```python
from build123d import *

# Parameters (mm, degrees)
F0_W     = 40
F0_H     = 20
F1_DEPTH = 20
F3_DEPTH = 4
F4_DEPTH = 2
F5_DEPTH = 2
F6_W     = 40
F6_H     = 2
F7_DEPTH = 3


with BuildPart() as f1:
    # F0 (on Top) → F1 (new body)
    with BuildSketch(Plane.XY):
        Rectangle(F0_W, F0_H)
    extrude(amount=F1_DEPTH)

    # F2 (on face) → F3 (join)
    with BuildSketch(Plane.XY.offset(20)):
        with BuildLine():
            Line((-10, -1.5), (-10, 1.5))
            ThreePointArc((-10, 1.5), (-11.5, 0), (-10, -1.5))
        make_face()
        with BuildLine():
            ThreePointArc((-8.5, 0), (-8.9393398282, 1.0606601718), (-10, 1.5))
            Line((-10, 1.5), (-10, -1.5))
            ThreePointArc((-10, -1.5), (-8.9393398282, -1.0606601718), (-8.5, 0))
        make_face()
        with BuildLine():
            Line((10, -1.5), (10, 1.5))
            ThreePointArc((10, 1.5), (8.5, 0), (10, -1.5))
        make_face()
        with BuildLine():
            ThreePointArc((11.5, 0), (11.0606601718, 1.0606601718), (10, 1.5))
            Line((10, 1.5), (10, -1.5))
            ThreePointArc((10, -1.5), (11.0606601718, -1.0606601718), (11.5, 0))
        make_face()
    extrude(amount=F3_DEPTH)

    # F4 (add): a face of the model
    f4_faces = [f1.faces().sort_by_distance(p)[0] for p in [
        (0, -10, 10),
    ]]
    extrude(f4_faces, amount=F4_DEPTH)

    # F5 (add): a face of the model
    f5_faces = [f1.faces().sort_by_distance(p)[0] for p in [
        (0, 10, 10),
    ]]
    extrude(f5_faces, amount=F5_DEPTH)

    # F6 (on face) → F7 (join)
    with BuildSketch(Plane(origin=(0, 0, 0), x_dir=(1, 0, 0), z_dir=(0, 0, -1))):
        with Locations((0, 11)):
            Rectangle(F6_W, F6_H)
        with Locations((0, -11)):
            Rectangle(F6_W, F6_H)
    extrude(amount=F7_DEPTH)


solid = f1.part
```
The model under review builds one solid part; all positions refer to its coordinate system, in mm. A direction names the side the tool comes from. Round coordinates to 2 decimals unless told otherwise and drop trailing zeros. Write each loop counter-clockwise with the first axis right and the second up, starting at its lowest first coordinate (ties: lowest second). Pieces come first, ordered by that corner, then holes. Notation, with made-up numbers: M -35.5,22 L -1.5,22 A16 ccw -1.5,43 Z; hole C 67.25,65 d10. An arc over 180 degrees is marked long. Use CSV: the item, a comma, the result in double quotes. Start each with the question number.
(1) For line 1 along Z through (x, y) = (0.5, 6.75); line 2 along Y through (x, z) = (-11, 20.5), list the stretches that pass through material, from the lowest coordinate up.
(2) We need section A-A, the plane x = 0. State the section outline as (y, z) points, then the cut area to 3 significant figures.
(3) Clearance check with flat-ended pins moving along their axes: P1, Ø3, axis at x = -5, y = 6, coming from the -Z side; P2, Ø8, axis at x = 15, y = 7.5, coming from the +Z side. State where each tip first meets the part, or that it passes through.
(4) Tool access review of faces 4 (the face through (0, -12, 9)), 5 (the face through (0, -10, -1)): name each direction out of +Z, -Z, +X, -X, +Y, -Y from which nothing blocks a thin tool from reaching the whole face with its end or side.
(5) We need section B-B, the plane y = 3. State the section outline as (x, z) points, then the cut area to 3 significant figures.
(6) We need section C-C, the plane x = 11. State the section outline as (y, z) points.
(7) The part is to be moulded in two halves that separate along Y. For faces 1 (the face through (0, 12, 8)), 2 (the face through (-20, 0, 9)), 3 (the face through (0, 10, -1)), say which applies: +Y half, -Y half, draft (parallel to the pull), parting line (faces both ways), or undercut.
Findings:
1,line 1,"0 to 20"
1,line 2,"-1.12 to 1.12"
2,outline,"M -12,-3 L -10,-3 L -10,0 L 10,0 L 10,-3 L 12,-3 L 12,20 L -12,20 Z"
2,area,"492 mm^2"
3,P1,"z = 0"
3,P2,"z = 20"
4,face 4,"+Z, -Z, +X, -X, -Y"
4,face 5,"-Z, +X, -X"
5,outline,"M -20,0 L 20,0 L 20,20 L -20,20 Z"
5,area,"800 mm^2"
6,outline,"M -12,-3 L -10,-3 L -10,0 L 10,0 L 10,-3 L 12,-3 L 12,20 L 1.12,20 L 1.12,24 L -1.12,24 L -1.12,20 L -12,20 Z"
7,face 1,"+Y half"
7,face 2,"draft"
7,face 3,"undercut"
